Design review of the part built by this model. Coordinates are the model's own, in mm. A direction names the side the tool comes from. Coordinates: 2 decimals unless noted, no trailing zeros. Write each loop counter-clockwise with the first axis right and the second up, starting at its lowest first coordinate (ties: lowest second). Pieces come first, ordered by that corner, then holes.
Q1. Clearance check with a flat-ended pin moving along its axis: pin 1 Ø1.5 at (x, z) = (-34.5, -14.5) entering from +Y. State where the tip first meets the part, or that it passes through.
Q2. To check wall thickness, follow probe 1 along X at (y, z) = (-2.4, -18.5); probe 2 along X at (y, z) = (-1.85, 25); probe 3 along X at (y, z) = (-4.5, 26.5). State the ranges of each line that lie inside material, in increasing order.
Q3. The part is to be moulded in two halves that separate along Z. For faces 1 (the face through (-1, -6, 0)), 2 (the face through (-31.1, -3, 25.5)), 3 (the face through (42.9, -2.96, -30.43)), say which applies: +Z half, -Z half, draft (parallel to the pull), parting line (faces both ways), or undercut.
Q4. Add section B-B, the plane y = -3.7. Give the boundary of the cut face in (x, z), plus the area to 3 significant figures.
Q5. Add section C-C, the plane z = -15. Give the boundary of the cut face in (x, y).
Q6. Add section A-A, the plane x = -31. Give the boundary of the cut face in (y, z).
Q7. Machinability: for faces 4 (the face through (-30.9, -3, 12.5)), 5 (the face through (42.93, -2.96, 30.4)), which of the approach directions +Z, -Z, +X, -X, +Y, -Y give a long, thin tool a straight path to every point of the face, cutting with its end or side? Answer none if there is none.
Q8. Add section D-D, the plane z = 16.5. Give the boundary of the cut face in (x, y), plus the area to 3 significant figures.
from build123d import *

# Parameters (mm, degrees)
F1_DEPTH = 6


with BuildPart() as f1:
    # F0 (on Front) → F1 (new body)
    with BuildSketch(Plane.XZ):
        with BuildLine():
            ThreePointArc((-43.5, -21), (-40.571068, -28.071068), (-33.5, -31))
            Line((-33.5, -31), (41.5, -31))
            ThreePointArc((41.5, -31), (42.914214, -30.414214), (43.5, -29))
            Line((43.5, -29), (43.5, 29))
            ThreePointArc((43.5, 29), (42.914214, 30.414214), (41.5, 31))
            Line((41.5, 31), (-33.5, 31))
            ThreePointArc((-33.5, 31), (-40.571068, 28.071068), (-43.5, 21))
            Line((-43.5, 21), (-43.5, -21))
        make_face()
        with BuildLine():
            ThreePointArc((-37, -18.5), (-31, -12.5), (-25, -18.5))
            Line((-25, -18.5), (-25, -19.5))
            ThreePointArc((-25, -19.5), (-31, -25.5), (-37, -19.5))
            Line((-37, -19.5), (-37, -18.5))
        make_face(mode=Mode.SUBTRACT)
        with BuildLine():
            ThreePointArc((-25, 18.5), (-31, 12.5), (-37, 18.5))
            Line((-37, 18.5), (-37, 19.5))
            ThreePointArc((-37, 19.5), (-31, 25.5), (-25, 19.5))
            Line((-25, 19.5), (-25, 18.5))
        make_face(mode=Mode.SUBTRACT)
    extrude(amount=F1_DEPTH)


solid = f1.part
Here are the results:
1. pin 1: stops at y = 0
2. probe 1: x = -43.5 to -37, -25 to 43.5
2. probe 2: x = -42.67 to -33.4, -28.6 to 43.5
2. probe 3: x = -41.85 to 43.5
3. face 1: draft
3. face 2: undercut
3. face 3: -Z half
4. outline: (-43.5, -21) arc R10 ccw to (-33.5, -31) - (41.5, -31) arc R2 ccw to (43.5, -29) - (43.5, 29) arc R2 ccw to (41.5, 31) - (-33.5, 31) arc R10 ccw to (-43.5, 21) - close; hole (-37, -19.5) arc R6 ccw to (-25, -19.5) - (-25, -18.5) arc R6 ccw to (-37, -18.5) - close; hole (-37, 18.5) arc R6 ccw to (-25, 18.5) - (-25, 19.5) arc R6 ccw to (-37, 19.5) - close
4. area: 5,100 mm2
5. outline: (-43.5, -6) - (-35.87, -6) - (-35.87, 0) - (-43.5, 0) - close; (-26.13, -6) - (43.5, -6) - (43.5, 0) - (-26.13, 0) - close
6. outline: (-6, -31) - (0, -31) - (0, -25.5) - (-6, -25.5) - close; (-6, -12.5) - (0, -12.5) - (0, 12.5) - (-6, 12.5) - close; (-6, 25.5) - (0, 25.5) - (0, 31) - (-6, 31) - close
7. face 4: +Y, -Y
7. face 5: +Z, +X, +Y, -Y
8. outline: (-43.5, -6) - (-36.66, -6) - (-36.66, 0) - (-43.5, 0) - close; (-25.34, -6) - (43.5, -6) - (43.5, 0) - (-25.34, 0) - close
8. area: 454 mm2
